Work out the finished part from the listing and answer in its coordinate system (mm). Face numbers are marked on the shaded views. A direction names the side the tool comes from. Round coordinates to 2 decimals unless told otherwise and drop trailing zeros. Write each loop counter-clockwise with the first axis right and the second up, starting at its lowest first coordinate (ties: lowest second). Pieces come first, ordered by that corner, then holes. Notation, with made-up numbers: (73, 53) -> (85, 53) arc R32 cw to (85, 92) -> close; hole circle Ø5 at (25.25, 43). An arc over 180 degrees is marked (long way). Answer as a JSON object with one key per item and string values. Group by question number.
from build123d import *

# Parameters (mm, degrees)
F0_W     = 25
F0_H     = 14
F0_R     = 3
F0_R_2   = 2.5
F1_DEPTH = 16
F2_R     = 1
F3_DEPTH = 25
F4_W     = 14
F4_H     = 10
F5_DEPTH = 25


with BuildPart() as f1:
    # F0 (on Front) → F1 (new body)
    with BuildSketch(Plane.XZ):
        Rectangle(F0_W, F0_H)
        with Locations((-7.5, 0)):
            Circle(F0_R, mode=Mode.SUBTRACT)
        with Locations((7.5, 0)):
            Circle(F0_R_2, mode=Mode.SUBTRACT)
    extrude(amount=F1_DEPTH)

    # F2 (on face) → F3 (cut)
    with BuildSketch(Plane.XY.offset(7)):
        with Locations((-5, -9)):
            Circle(F2_R)
    extrude(amount=-F3_DEPTH, mode=Mode.SUBTRACT)

    # F4 (on face) → F5 (cut)
    with BuildSketch(Plane(origin=(-12.5, 0, 0), x_dir=(0, -1, 0), z_dir=(-1, 0, 0))):
        with Locations((9, 0)):
            Rectangle(F4_W, F4_H)
    extrude(amount=-F5_DEPTH, mode=Mode.SUBTRACT)


solid = f1.part
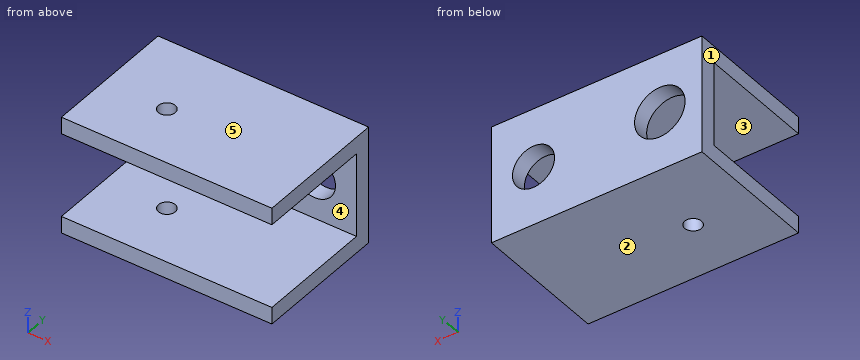
1) A cutting plane is placed at A-A on z = 0. Determine the outline of the cut face in (x, y), plus the area to 3 significant figures.
2) A cutting plane is placed at D-D on y = -1.25. Determine the outline of the cut face in (x, z), plus the area to 3 significant figures.
3) Straight lines are drawn through the part: L1, parallel to X at y = -0.5, z = 0; L2, parallel to Z at x = -3, y = -12.5; L3, parallel to Z at x = -7.5, y = -0.8. For each, find the intervals that lie inside material, in ascending order.
4) For a pull along Z with two mould halves and no side action, classify the marked faces 1, 2 and 3 as released by +Z, released by -Z, zero draft, split by the parting line, or undercut.
5) Each of these flat-tipped pins is pushed along its axis until it touches: P1, Ø3, axis at x = -5, y = -9, coming from the -Z side; P2, Ø5, axis at x = -4, z = -0.5, coming from the -Y side. Where does it stop, or does it pass through?
6) A tool of negligible diameter and unlimited length cuts with its end or side. For the marked faces 4 and 5, from which of +Z, -Z, +X, -X, +Y, -Y can it reach the whole face along a straight path? Write none if from no direction.
7) A cutting plane is placed at B-B on x = 7.5. Determine the outline of the cut face in (y, z).
8) A cutting plane is placed at C-C on y = -5.5. Determine the outline of the cut face in (x, z), plus the area to 3 significant figures.
Established:
{
 "1": {"outline": "(-12.5, -2) -> (-10.5, -2) -> (-10.5, 0) -> (-12.5, 0) -> close; (-4.5, -2) -> (5, -2) -> (5, 0) -> (-4.5, 0) -> close; (10, -2) -> (12.5, -2) -> (12.5, 0) -> (10, 0) -> close", "area": "28.0 mm²"},
 "2": {"outline": "(-12.5, -7) -> (12.5, -7) -> (12.5, 7) -> (-12.5, 7) -> close; hole circle Ø6 at (-7.5, 0); hole circle Ø5 at (7.5, 0)", "area": "302 mm²"},
 "3": {"L1": "x = -12.5 to -10.5, -4.5 to 5, 10 to 12.5", "L2": "z = -7 to -5, 5 to 7", "L3": "z = -7 to -3, 3 to 7"},
 "4": {"face 1": "zero draft", "face 2": "released by -Z", "face 3": "undercut"},
 "5": {"P1": "stops at z = -7", "P2": "stops at y = -2"},
 "6": {"face 4": "+X, -X, -Y", "face 5": "+Z, +X, -X, +Y, -Y"},
 "7": {"outline": "(-16, -7) -> (0, -7) -> (0, -2.5) -> (-2, -2.5) -> (-2, -5) -> (-16, -5) -> close; (-16, 5) -> (-2, 5) -> (-2, 2.5) -> (0, 2.5) -> (0, 7) -> (-16, 7) -> close"},
 "8": {"outline": "(-12.5, -7) -> (12.5, -7) -> (12.5, -5) -> (-12.5, -5) -> close; (-12.5, 5) -> (12.5, 5) -> (12.5, 7) -> (-12.5, 7) -> close", "area": "100 mm²"}
}
